Design review of the part built by this model. Coordinates are the model's own, in mm. Face numbers are marked on the shaded views. A direction names the side the tool comes from. Coordinates: 2 decimals unless noted, no trailing zeros. Order: outer loops, then holes, each group sorted by start corner. A loop starts at its lowest first (then second) coordinate and runs counter-clockwise, first axis right, second up. Notation, with made-up numbers: M 6.25,-38 L 59.25,-38 A17 ccw 59.25,-12 Z; hole C -22,42.25 d1. An arc over 180 degrees is marked long. Answer as a JSON object with one key per item and string values.
from build123d import *

# Parameters (mm, degrees)
F0_R      = 12.7
F1_DEPTH  = 30.1625
F2_R      = 7.874
F3_R      = 2.54
F4_DEPTH  = 30.1625
F5_DEPTH  = 19.05
F6_DEPTH  = 41.275
F8_R      = 2.54
F9_R      = 6.35
F10_DEPTH = 22.353
F11_W     = 59.1995969771
F11_H     = 22.3266
F12_DEPTH = 34.799
F13_DEPTH = 45.212


with BuildPart() as f1:
    # F0 (on Front) → F1 (new body, symmetric)
    with BuildSketch(Plane.XZ):
        with BuildLine():
            Line((85.852, 0), (22.352, 0))
            ThreePointArc((22.352, 0), (-15.8052507731, 15.8052507731), (0, -22.352))
            Line((0, -22.352), (91.8464, -22.352))
            Line((91.8464, -22.352), (85.852, 0))
        make_face()
        Circle(F0_R, mode=Mode.SUBTRACT)
    extrude(amount=F1_DEPTH, both=True)

    # F3
    f3_edges = [f1.edges().sort_by_distance(p)[0] for p in [
        (22.352, 0, 0),
    ]]
    fillet(f3_edges, radius=F3_R)


with BuildPart() as f1b:
    # F0 (on Front) → F1, piece 2 (new body, symmetric)
    with BuildSketch(Plane.XZ):
        Polygon((150.0886, 0), (117.2464, 0), (117.2464, -22.352), (194.2084, -22.352), (194.2084, 0), align=None)
    extrude(amount=F1_DEPTH, both=True)

    # F2
    f2_edges = [f1b.edges().sort_by_distance(p)[0] for p in [
        (194.2084, 0, 0),
    ]]
    fillet(f2_edges, radius=F2_R)


with BuildPart() as f4:
    # F0 (on Front) → F4 (new body, symmetric)
    with BuildSketch(Plane.XZ):
        Polygon((117.2464, 0), (85.852, 0), (91.8464, -22.352), (117.2464, -22.352), align=None)
    extrude(amount=F4_DEPTH, both=True)

    # F5 (cut): a face of the model
    f5_faces = [f4.faces().sort_by_distance(p)[0] for p in [
        (102.995076446, -30.1625, -10.7828073942),
    ]]
    extrude(f5_faces, amount=-F5_DEPTH, mode=Mode.SUBTRACT)


with BuildPart() as f4b:
    # F0 (on Front) → F4, piece 2 (new body, symmetric)
    with BuildSketch(Plane.XZ):
        with BuildLine():
            ThreePointArc((131.0386, 34.798), (127.4644153616, 16.0823576341), (117.2464, 0))
            Line((117.2464, 0), (150.0886, 0))
            Line((150.0886, 0), (150.0886, 34.798))
            Line((150.0886, 34.798), (131.0386, 34.798))
        make_face()
    extrude(amount=F4_DEPTH, both=True)

    # F6 (cut): a face of the model
    f6_faces = [f4b.faces().sort_by_distance(p)[0] for p in [
        (138.0621984193, 30.1625, 15.7456064231),
    ]]
    extrude(f6_faces, amount=-F6_DEPTH, mode=Mode.SUBTRACT)


with BuildPart() as f1b_1:
    add(f1b.part)

    # F7: union F4, F1, F4b
    add(f4.part)
    add(f1.part)
    add(f4b.part)

    # F8
    f8_edges = [f1b_1.edges().sort_by_distance(p)[0] for p in [
        (150.0886, -20.6375, 34.798),
        (150.0886, -20.6375, 0),
    ]]
    fillet(f8_edges, radius=F8_R)

    # F9 (on face) → F10 (cut, through all)
    with BuildSketch(Plane.XY):
        with Locations((155.3464, 7.8105)):
            Circle(F9_R)
    extrude(amount=-F10_DEPTH, mode=Mode.SUBTRACT)

    # F11 (on Top) → F12 (cut, through all)
    with BuildSketch(Plane.XY):
        with Locations((-0.0117294312, 0)):
            Rectangle(F11_W, F11_H)
    extrude(amount=F12_DEPTH, mode=Mode.SUBTRACT)

    # F11 (on Top) → F13 (cut)
    with BuildSketch(Plane.XY):
        with Locations((-0.0117294312, 0)):
            Rectangle(F11_W, F11_H)
    extrude(amount=-F13_DEPTH, mode=Mode.SUBTRACT)


solid = f1b_1.part
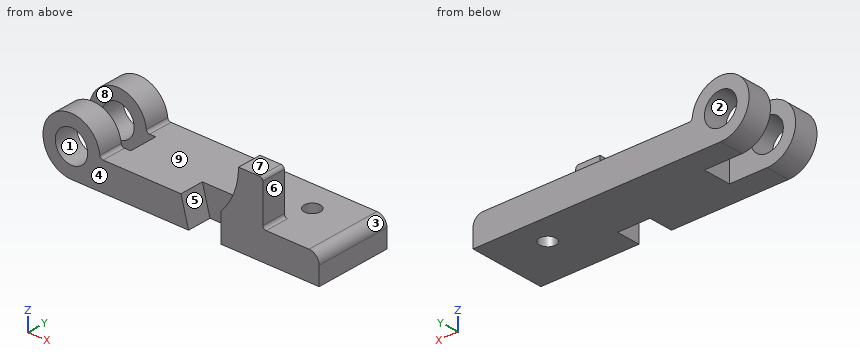
1) Tool access review of the marked faces 5, 6, 7, 8 and 9: name each direction out of +Z, -Z, +X, -X, +Y, -Y from which nothing blocks a thin tool from reaching the whole face with its end or side.
Taken from the geometry:
{"face 5": "+Z, -Y", "face 6": "+Z, +X, +Y, -Y", "face 7": "+Z, +X, -X, +Y, -Y", "face 8": "+Z, -Z, -X", "face 9": "+Z, +Y"}
2) Mouldability with a two-part tool opening along Z and no side actions: class the marked faces 1, 2, 3 and 4 as released by +Z, released by -Z, zero draft, split by the parting line, or undercut.
Taken from the geometry:
{"face 1": "undercut", "face 2": "undercut", "face 3": "released by +Z", "face 4": "zero draft"}
3) Add section C-C (y = 24). State the section outline as (x, z) points, and give its area (3 significant figures).
Taken from the geometry:
{"outline": "M 0,-22.35 L 194.21,-22.35 L 194.21,-7.87 A7.87 ccw 186.33,0 L 24.76,0 A2.54 cw 22.24,2.28 A22.35 ccw long Z; hole C 0,0 d25.4", "area": "5,000 mm2"}
4) Add section A-A (y = -21). State the section outline as (x, z) points, and give its area (3 significant figures).
Taken from the geometry:
{"outline": "M 0,-22.35 L 91.85,-22.35 L 85.85,0 L 24.76,0 A2.54 cw 22.24,2.28 A22.35 ccw long Z; M 117.25,-22.35 L 194.21,-22.35 L 194.21,-7.87 A7.87 ccw 186.33,0 L 152.63,0 A2.54 cw 150.09,2.54 L 150.09,32.26 A2.54 ccw 147.55,34.8 L 131.04,34.8 A50.8 cw 117.25,0 Z; hole C 0,0 d25.4", "area": "5,180 mm2"}
5) Insertion check: pin 1 Ø12 at (x, y) = (33.5, 13.5) entering from +Z; pin 2 Ø10.5 at (x, z) = (126.5, 9) entering from +Y; pin 3 Ø15 at (y, z) = (-20.5, 19.5) entering from +X. Each pin has a flat end and moves straight along its axis. Give the tip position at first contact, or say it passes through.
Taken from the geometry:
{"pin 1": "stops at z = 0", "pin 2": "stops at y = -11.11", "pin 3": "stops at x = 150.09"}
6) Add section D-D (x = 9). State the section outline as (y, z) points, and give its area (3 significant figures).
Taken from the geometry:
{"outline": "M -30.16,-22.35 L -11.16,-22.35 L -11.16,-8.96 L -30.16,-8.96 Z; M -30.16,8.96 L -11.16,8.96 L -11.16,20.46 L -30.16,20.46 Z; M 11.16,-22.35 L 30.16,-22.35 L 30.16,-8.96 L 11.16,-8.96 Z; M 11.16,8.96 L 30.16,8.96 L 30.16,20.46 L 11.16,20.46 Z", "area": "946 mm2"}
7) Add section B-B (z = -4). State the section outline as (x, y) points.
Taken from the geometry:
{"outline": "M -21.99,-30.16 L -12.05,-30.16 L -12.05,-11.16 L -21.99,-11.16 Z; M -21.99,11.16 L -12.05,11.16 L -12.05,30.16 L -21.99,30.16 Z; M 12.05,-30.16 L 86.92,-30.16 L 86.92,-11.11 L 117.25,-11.11 L 117.25,-30.16 L 193.19,-30.16 L 193.19,30.16 L 12.05,30.16 L 12.05,11.16 L 29.59,11.16 L 29.59,-11.16 L 12.05,-11.16 Z; hole C 155.35,7.81 d12.7"}
8) To check wall thickness, follow L1, parallel to Y at x = 23, z = -7; L2, parallel to Z at x = 0, y = -25; L3, parallel to Z at x = 46, y = -26. State the ranges of each line that lie inside material, in increasing order.
Taken from the geometry:
{"L1": "y = -30.16 to -11.16, 11.16 to 30.16", "L2": "z = -22.35 to -12.7, 12.7 to 22.35", "L3": "z = -22.35 to 0"}
